```python
from build123d import *
from build123d import SkipClean  # not in build123d's __all__

# Parameters (mm, degrees)
F1_DEPTH = 99.8
F2_R     = 2.875
F3_DEPTH = 4
F4_DEPTH = 2
F6_DEPTH = 2


with BuildPart() as f1:
    # F0 (on Top) → F1 (new body)
    with BuildSketch(Plane.XY):
        with BuildLine():
            ThreePointArc((-17.2717254494, 8.5), (-16.8769277982, 9.2591472661), (-16.4487841496, 10))
            Line((-16.4487841496, 10), (-19.25, 10))
            Line((-19.25, 10), (-20.572897503, 9.5070659068))
            Line((-20.572897503, 9.5070659068), (-23.85, 3))
            Line((-23.85, 3), (-23.85, -3))
            Line((-23.85, -3), (-20.572897503, -9.5070659068))
            Line((-20.572897503, -9.5070659068), (-19.25, -10))
            Line((-19.25, -10), (-16.4487841496, -10))
            ThreePointArc((-16.4487841496, -10), (-16.8769277982, -9.2591472661), (-17.2717254494, -8.5))
            Line((-17.2717254494, -8.5), (-19.25, -8.5))
            Line((-19.25, -8.5), (-22.35, -3))
            Line((-22.35, -3), (-22.35, 0))
            Line((-22.35, 0), (-22.35, 3))
            Line((-22.35, 3), (-19.25, 8.5))
            Line((-19.25, 8.5), (-17.2717254494, 8.5))
        make_face()
    extrude(amount=F1_DEPTH)

    # F2 (on face) → F3 (cut)
    with BuildSketch(Plane(origin=(-23.85, 0, 0), x_dir=(0, -1, 0), z_dir=(-1, 0, 0))):
        with Locations((0, 14.26)):
            Circle(F2_R)
        with Locations((0, 28.52)):
            Circle(F2_R)
        with Locations((0, 42.78)):
            Circle(F2_R)
        with Locations((0, 57.04)):
            Circle(F2_R)
        with Locations((0, 71.3)):
            Circle(F2_R)
        with Locations((0, 85.56)):
            Circle(F2_R)
    extrude(amount=-F3_DEPTH, mode=Mode.SUBTRACT)

    # F0 (on Top) → F4 (join)
    with BuildSketch(Plane.XY):
        with BuildLine():
            ThreePointArc((-17.2717254494, -8.5), (-19.25, 0), (-17.2717254494, 8.5))
            Line((-17.2717254494, 8.5), (-19.25, 8.5))
            Line((-19.25, 8.5), (-22.35, 3))
            Line((-22.35, 3), (-22.35, 0))
            Line((-22.35, 0), (-22.35, -3))
            Line((-22.35, -3), (-19.25, -8.5))
            Line((-19.25, -8.5), (-17.2717254494, -8.5))
        make_face()
    extrude(amount=F4_DEPTH)

    # F5 (on face) → F6 (join)
    with BuildSketch(Plane.XY.offset(99.8)):
        with BuildLine():
            ThreePointArc((-17.2717254494, -8.5), (-19.25, 0), (-17.2717254494, 8.5))
            Line((-17.2717254494, 8.5), (-19.25, 8.5))
            Line((-19.25, 8.5), (-22.35, 3))
            Line((-22.35, 3), (-22.35, -3))
            Line((-22.35, -3), (-19.25, -8.5))
            Line((-19.25, -8.5), (-17.2717254494, -8.5))
        make_face()
    with SkipClean():  # cleaning this boolean's faces spoils the solid; the shape is the same uncleaned
        extrude(amount=-F6_DEPTH)


solid = f1.part
```
Check sheet for the modelled part. Datum: model origin and axes. Units: mm. A direction names the side the tool comes from. Give positions to 0.01 mm unless a question says otherwise; leave off trailing zeros. Loops run counter-clockwise (first coordinate to the right, second up) from the corner with the lowest first, then second, coordinate; pieces in that order, holes last. Notation, with made-up numbers: (72, -1.5) - (121, -1.5) arc R21 cw to (121, 18.5) - close; hole circle Ø6 at (-32, -7.5). An arc over 180 degrees is marked (long way). One line per question, with ' | ' between items. Start each with the question number.
1. Draft check along Z on faces 1 (the flat face through (-20.778, -5.788, 49.229)), 2 (the flat face through (-18, -10, 49)), 3 (the flat face through (-21, 0, 0)), 4 (the cylindrical face through (-23.11, 0.623, 39.973)). Enter one of: released by +Z, released by -Z, zero draft, split by the parting line, or undercut.
2. Gauge pin test, flat ends, axial feed: pin 1 Ø6.5 at (y, z) = (0.5, 71) entering from +X; pin 2 Ø1.5 at (x, z) = (-22.5, 61.5) entering from +Y; pin 3 Ø3.5 at (y, z) = (0, 57.04) entering from +X. Record the tip position at first contact, or that the pin passes through.
3. Cross-section at D-D, the plane y = -4. Enter the section's corners in (x, z).
4. Cross-section at C-C, the plane z = 80. Enter the section's corners in (x, y).
5. Set-up check for faces 5 (the flat face through (-20.822, 5.712, 49.229)), 6 (the cylindrical face through (-23.11, 0.623, 54.233)): record each of +Z, -Z, +X, -X, +Y, -Y from which the full face is reachable in a straight line by a thin tool's end or side.
6. Cross-section at A-A, the plane y = 0. Give the number of separate pieces and of enclosed holes in the cut face, plus the area to 3 significant figures.
7. Material ranges on line 1 along X through (y, z) = (3, 6.5); line 2 along Y through (x, z) = (-19, 23.5), recorded low to high. Write a range as [from, to].
8. Cross-section at B-B, the plane z = 42.78. Enter the section's corners in (x, y) (3 decimals), plus the area to 3 significant figures.
Check result:
1) face 1: undercut | face 2: zero draft | face 3: released by -Z | face 4: undercut
2) pin 1: stops at x = -21.93 | pin 2: stops at y = 7.17 | pin 3: passes through
3) outline: (-23.35, 0) - (-18.83, 0) - (-18.83, 2) - (-21.79, 2) - (-21.79, 97.8) - (-18.83, 97.8) - (-18.83, 99.8) - (-23.35, 99.8) - close
4) outline: (-23.85, -3) - (-20.57, -9.51) - (-19.25, -10) - (-16.45, -10) arc R19.25 cw to (-17.27, -8.5) - (-19.25, -8.5) - (-22.35, -3) - (-22.35, 3) - (-19.25, 8.5) - (-17.27, 8.5) arc R19.25 cw to (-16.45, 10) - (-19.25, 10) - (-20.57, 9.51) - (-23.85, 3) - close
5) face 5: +X | face 6: +X, -X
6) separate pieces: 7 | enclosed holes: 0 | area: 110 mm2
7) line 1: x = [-23.85, -22.35] | line 2: y = [-10, -8.5], [8.5, 10]
8) outline: (-23.85, -3) - (-20.573, -9.507) - (-19.25, -10) - (-16.449, -10) arc R19.25 cw to (-17.272, -8.5) - (-19.25, -8.5) - (-22.35, -3) - (-22.35, -2.875) - (-23.85, -2.875) - close; (-23.85, 2.875) - (-22.35, 2.875) - (-22.35, 3) - (-19.25, 8.5) - (-17.272, 8.5) arc R19.25 cw to (-16.449, 10) - (-19.25, 10) - (-20.573, 9.507) - (-23.85, 3) - close | area: 29.6 mm2
